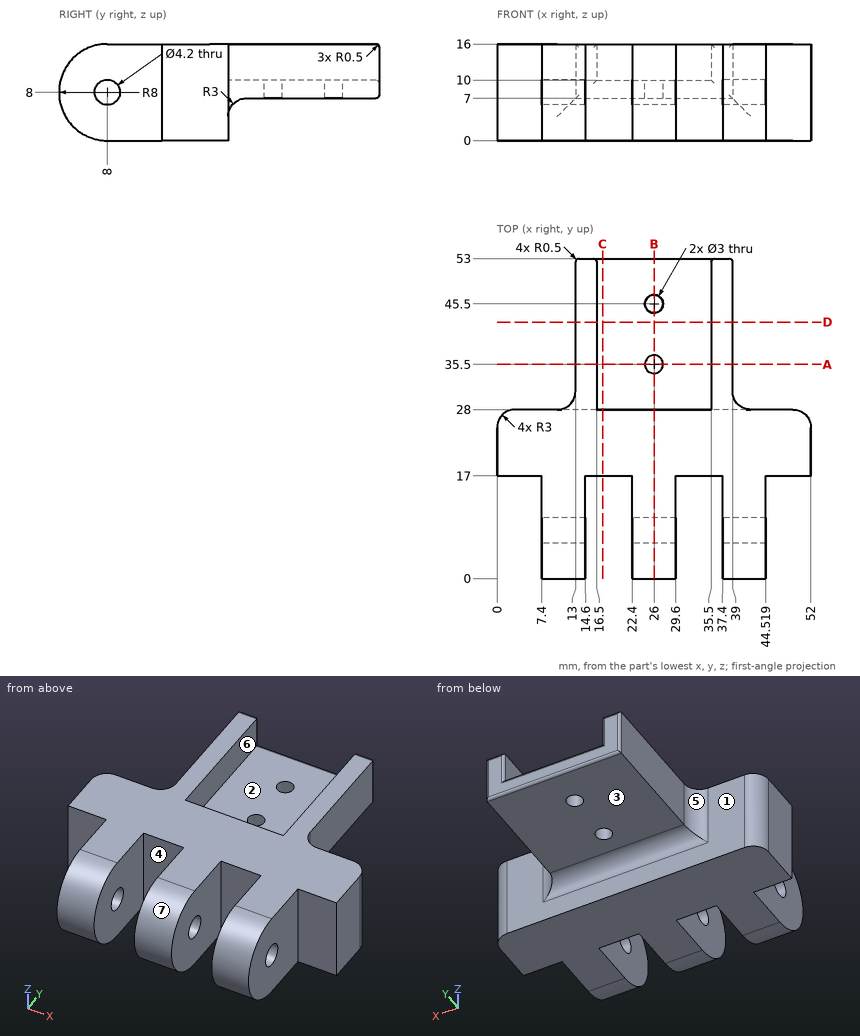
For this review, use the dimensioned drawing (mm, ordinates from the lowest corner) and the shaded views. A direction names the side the tool comes from. Round coordinates to 2 decimals unless told otherwise and drop trailing zeros. Write each loop counter-clockwise with the first axis right and the second up, starting at its lowest first coordinate (ties: lowest second). Pieces come first, ordered by that corner, then holes. Notation, with made-up numbers: (28, 37) - (72, 37) arc R15 ccw to (72, 42) - close; hole circle Ø3 at (-39, 13). An arc over 180 degrees is marked (long way). Use a Markdown table: item, result.
Q1. We need section D-D (y = 42.5). Give the boundary of the cut face in (x, z), plus the area to 3 significant figures.
Derived:
| item | result |
|---|---|
| outline | (13, 7) - (39, 7) - (39, 16) - (35.5, 16) - (35.5, 10) - (16.5, 10) - (16.5, 16) - (13, 16) - close |
| area | 120 mm2 |
Q2. We need section A-A (y = 35.5). Give the boundary of the cut face in (x, z).
Derived:
| item | result |
|---|---|
| outline | (13, 7) - (24.5, 7) - (24.5, 10) - (16.5, 10) - (16.5, 16) - (13, 16) - close; (27.5, 7) - (39, 7) - (39, 16) - (35.5, 16) - (35.5, 10) - (27.5, 10) - close |
Q3. We need section C-C (x = 17.5). Give the boundary of the cut face in (y, z).
Derived:
| item | result |
|---|---|
| outline | (17, 0) - (28, 0) - (28, 4) arc R3 cw to (31, 7) - (52.5, 7) arc R0.5 ccw to (53, 7.5) - (53, 9.5) arc R0.5 ccw to (52.5, 10) - (28, 10) - (28, 16) - (17, 16) - close |
Q4. The part is to be moulded in two halves that separate along X. For the marked faces 5, 6 and 7, say which applies: pulls with the +X half, pulls with the -X half, needs draft (parallel to the pull), parting line crosses it, or undercut.
Derived:
| item | result |
|---|---|
| face 5 | pulls with the -X half |
| face 6 | undercut |
| face 7 | needs draft |
Q5. Clearance check with flat-ended pins moving along their axes: pin 1 (5 mm diameter, centred on y = 37.5, z = 14.5, fed in from +X); pin 2 (8 mm diameter, centred on y = 8.5, z = 8.5, fed in from -X); pin 3 (8 mm diameter, centred on y = 7, z = 5, fed in from +X). State where each tip first meets the part, or that it passes through.
Derived:
| item | result |
|---|---|
| pin 1 | stops at x = 39 |
| pin 2 | stops at x = 7.4 |
| pin 3 | stops at x = 44.52 |
Q6. Machinability: for the marked faces 1, 2, 3 and 4, which of the approach directions +Z, -Z, +X, -X, +Y, -Y give a long, thin tool a straight path to every point of the face, cutting with its end or side? Answer none if there is none.
Derived:
| item | result |
|---|---|
| face 1 | -Z, +Y |
| face 2 | +Z, +Y |
| face 3 | -Z, +X, -X, +Y |
| face 4 | +Z, -Z, -Y |
Q7. Wall thickness on line 1 along X through (y, z) = (5, 5.5); line 2 along Y through (x, z) = (26, 8); line 3 along X through (y, z) = (47, 12.5): over which ranges is each line inside the solid? List them lowest first.
Derived:
| item | result |
|---|---|
| line 1 | x = 7.4 to 14.6, 22.4 to 29.6, 37.4 to 44.52 |
| line 2 | y = 0 to 5.9, 10.1 to 34, 37 to 44, 47 to 53 |
| line 3 | x = 13 to 16.5, 35.5 to 39 |
Q8. We need section B-B (x = 26). Give the boundary of the cut face in (y, z), plus the area to 4 significant figures.
Derived:
| item | result |
|---|---|
| outline | (8, 0) - (28, 0) - (28, 4) arc R3 cw to (31, 7) - (34, 7) - (34, 10) - (28, 10) - (28, 16) - (8, 16) arc R8 ccw to start; (37, 7) - (44, 7) - (44, 10) - (37, 10) - close; (47, 7) - (52.5, 7) arc R0.5 ccw to (53, 7.5) - (53, 9.5) arc R0.5 ccw to (52.5, 10) - (47, 10) - close; hole circle Ø4.2 at (8, 8) |
| area | 465.5 mm2 |
